Drawing for the job (mm, zero at the part's lowest x, y, z). A direction names the side the tool comes from. Give positions to 0.01 mm unless a question says otherwise; leave off trailing zeros. Write each loop counter-clockwise with the first axis right and the second up, starting at its lowest first coordinate (ties: lowest second). Pieces come first, ordered by that corner, then holes.
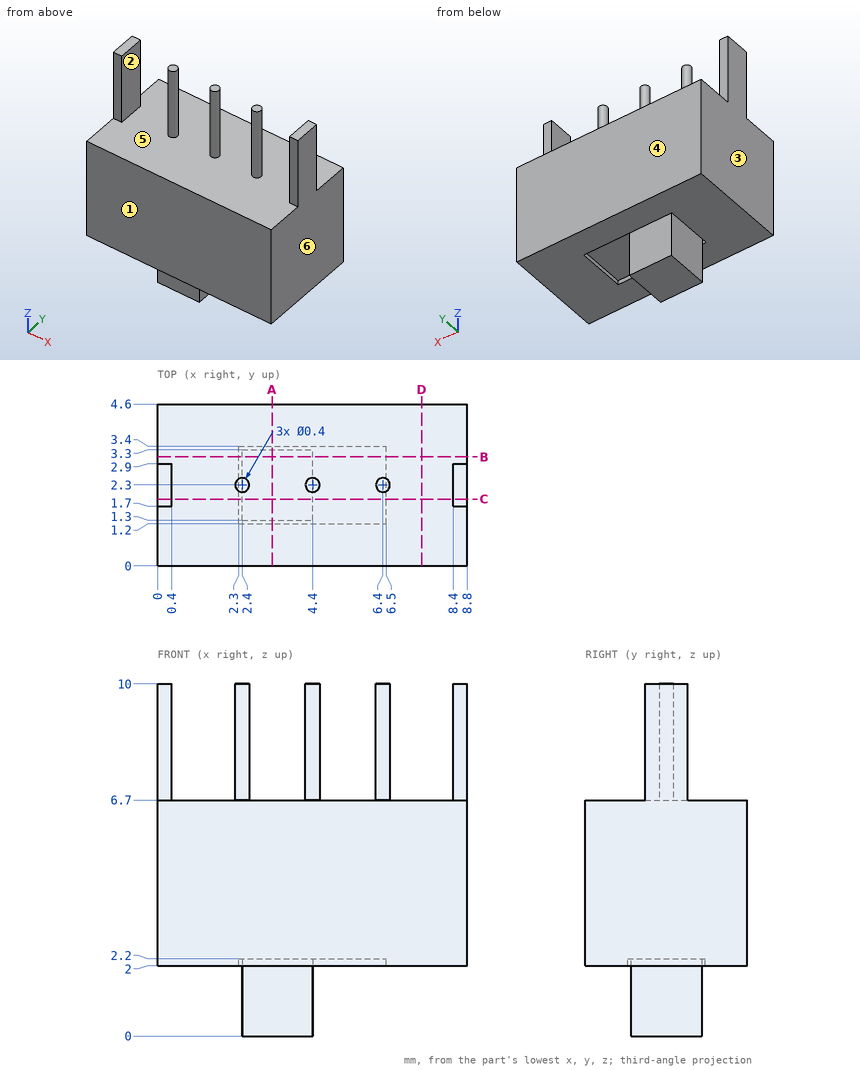
1. Slice it at D-D, the plane x = 7.5. Write the cut outline in (y, z), and give its area (3 significant figures).
Calculated:
outline: (0, 2) - (4.6, 2) - (4.6, 6.7) - (0, 6.7) - close
area: 21.6 mm2
2. Which spindle directions (+Z, -Z, +X, -X, +Y, -Y) get a long thin tool onto all of the face, cutting with end or side? Do the marked faces 1 and 2. Say none if no direction does.
Calculated:
face 1: +Z, -Z, +X, -X, -Y
face 2: +Z, +Y, -Y
3. Slice it at A-A, the plane x = 3.25. Write the cut outline in (y, z).
Calculated:
outline: (0, 2) - (1.2, 2) - (1.2, 2.2) - (1.3, 2.2) - (1.3, 0) - (3.3, 0) - (3.3, 2.2) - (3.4, 2.2) - (3.4, 2) - (4.6, 2) - (4.6, 6.7) - (0, 6.7) - close
4. Pin check, flat tips, straight feed: P1, Ø1.6, axis at x = 3, z = 0.5, coming from the +Y side; P2, Ø1, axis at y = 2, z = 0.5, coming from the +X side; P3, Ø0.6, axis at y = 2.5, z = 0.5, coming from the -X side. Stop position of each tip, or through.
Calculated:
P1: stops at y = 3.3
P2: stops at x = 4.4
P3: stops at x = 2.4
5. Slice it at B-B, the plane y = 3.1. Write the cut outline in (x, z).
Calculated:
outline: (0, 2) - (2.3, 2) - (2.3, 2.2) - (2.4, 2.2) - (2.4, 0) - (4.4, 0) - (4.4, 2.2) - (6.5, 2.2) - (6.5, 2) - (8.8, 2) - (8.8, 6.7) - (0, 6.7) - close
6. Pull direction X, two halves, no side cores. Call the marked faces 3, 4, 5 and 6: +X half, -X half, draft (parallel to the pull), parting line (faces both ways), or undercut.
Calculated:
face 3: -X half
face 4: draft
face 5: undercut
face 6: +X half
7. Probe probe 1 along X at (y, z) = (2.6, 8.5); probe 2 along X at (y, z) = (2.4, 7); probe 3 along Z at (x, y) = (0.5, 4.4). List the from-to ranges inside material, lowest first.
Calculated:
probe 1: x = 0 to 0.4, 8.4 to 8.8
probe 2: x = 0 to 0.4, 2.23 to 2.57, 4.23 to 4.57, 6.23 to 6.57, 8.4 to 8.8
probe 3: z = 2 to 6.7
8. Slice it at C-C, the plane y = 1.9. Write the cut outline in (x, z).
Calculated:
outline: (0, 2) - (2.3, 2) - (2.3, 2.2) - (2.4, 2.2) - (2.4, 0) - (4.4, 0) - (4.4, 2.2) - (6.5, 2.2) - (6.5, 2) - (8.8, 2) - (8.8, 10) - (8.4, 10) - (8.4, 6.7) - (0.4, 6.7) - (0.4, 10) - (0, 10) - close
